The figure shows three views and two pictorial views of one solid part (mm, origin at its lowest corner). Answer the questions. Give positions to 0.01 mm unless a question says otherwise; leave off trailing zeros. Order: outer loops, then holes, each group sorted by start corner. A loop starts at its lowest first (then second) coordinate and runs counter-clockwise, first axis right, second up. Notation, with made-up numbers: (59, -31) - (87, -31) arc R18 ccw to (87, -18) - close; hole circle Ø1 at (32.25, 38). An arc over 180 degrees is marked (long way). Use a Markdown table: item, result. Add a question column.
1. A cutting plane is placed at A-A on z = 3.25. Determine the outline of the cut face in (x, y) (1 decimal).
2. Consider L1, parallel to Y at x = 199.5, z = 3.5 (1 decimal); L2, parallel to Y at x = 272, z = 5.5 (1 decimal); L3, parallel to Y at x = 168, z = 2.25 (1 decimal). Determine where each line is inside the solid, lowest interval first.
3. A cutting plane is placed at B-B on x = 180. Determine the outline of the cut face in (y, z), and give its area (3 significant figures).
4. Flat-ended cylindrical pins translate along their axes: P1, Ø3, axis at x = 96, z = 4.5, coming from the +Y side; P2, Ø1.5, axis at x = 251.5, z = 2, coming from the +Y side (1 decimal); P3, Ø3, axis at y = 177, z = 1.5, coming from the +X side (1 decimal). Find the tip coordinate at first contact, or state that the pin passes through.
5. A cutting plane is placed at C-C on y = 192. Determine the outline of the cut face in (x, z).
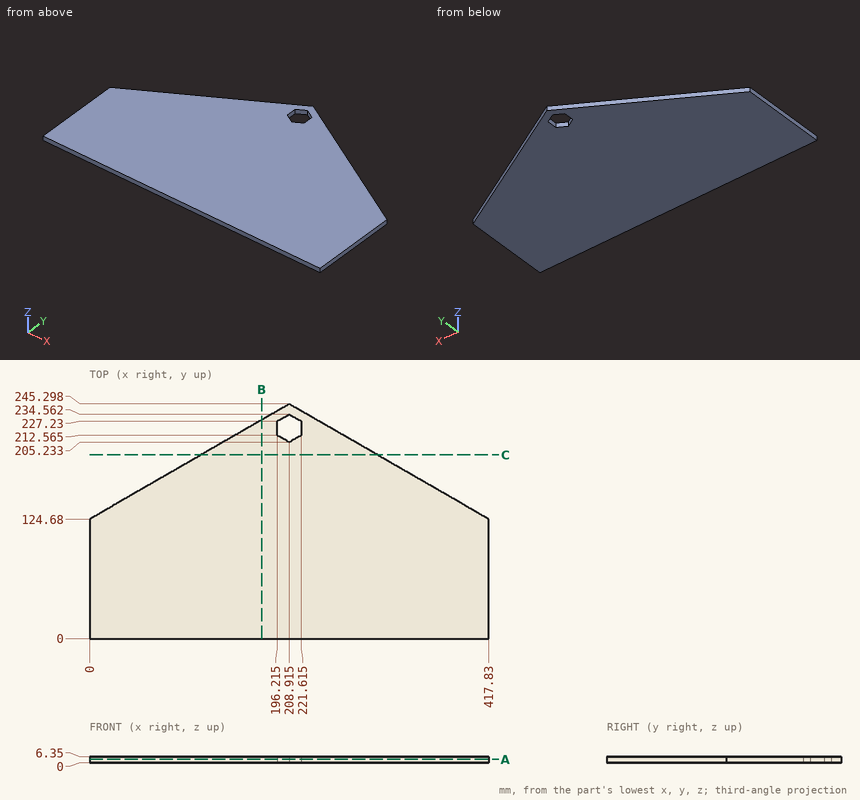
Output values:
| question | item | result |
|---|---|---|
| 1 | outline | (0, 0) - (417.8, 0) - (417.8, 124.7) - (208.9, 245.3) - (0, 124.7) - close; hole (196.2, 212.6) - (208.9, 205.2) - (221.6, 212.6) - (221.6, 227.2) - (208.9, 234.6) - (196.2, 227.2) - close |
| 2 | L1 | 0 to 210.7, 229.1 to 239.9 |
| 2 | L2 | 0 to 208.9 |
| 2 | L3 | 0 to 221.7 |
| 3 | outline | (0, 0) - (228.6, 0) - (228.6, 6.35) - (0, 6.35) - close |
| 3 | area | 1,450 mm² |
| 4 | P1 | y = 180.97 |
| 4 | P2 | y = 221.1 |
| 4 | P3 | x = 329.8 |
| 5 | outline | (116.6, 0) - (301.23, 0) - (301.23, 6.35) - (116.6, 6.35) - close |
